Can you work these out from the drawing? Everything is in mm from the part's minimum corner. A direction names the side the tool comes from. Give positions to 0.01 mm unless a question says otherwise; leave off trailing zeros. Write each loop counter-clockwise with the first axis right and the second up, starting at its lowest first coordinate (ties: lowest second). Pieces come first, ordered by that corner, then holes. Notation, with made-up numbers: M 45.5,-20.75 L 70.5,-20.75 A28 ccw 70.5,18.25 Z; hole C -20,-17.75 d1. An arc over 180 degrees is marked long. One line per item, written item: value.
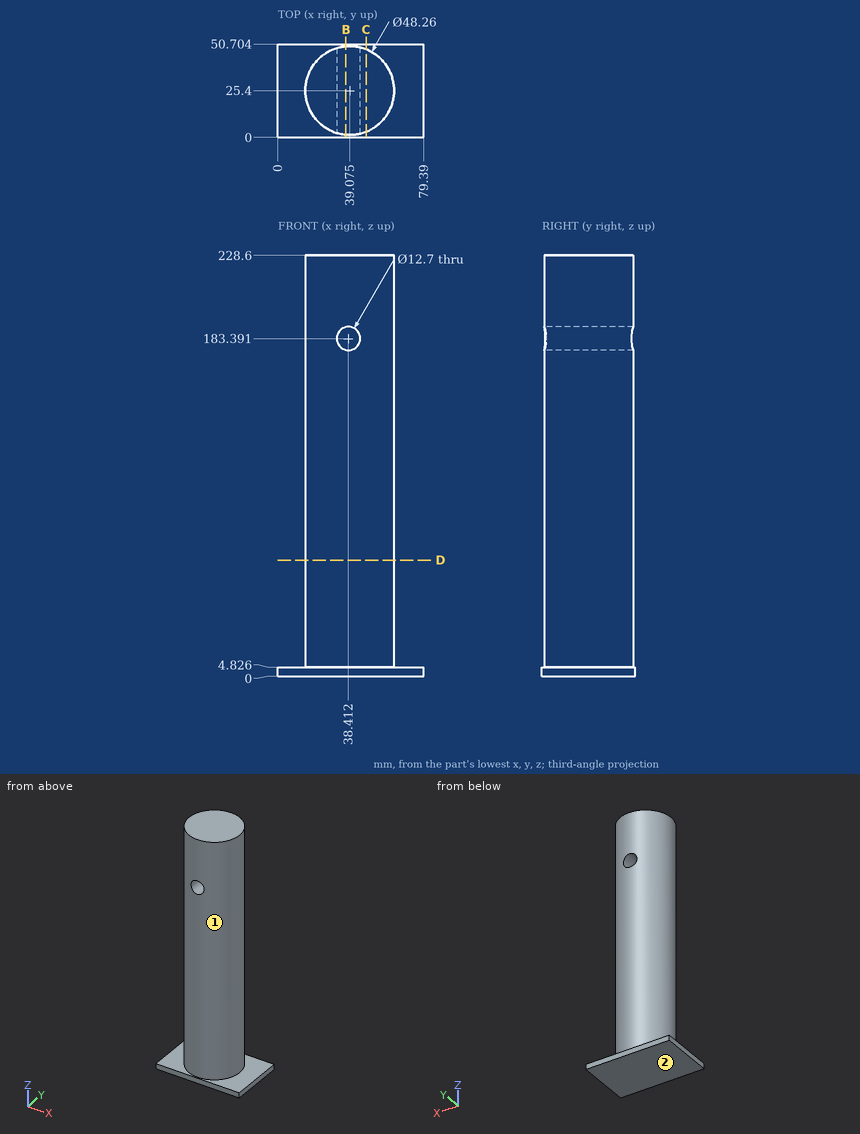
1) I'm going to push flat-ended pins straight in: pin 1 (6 mm diameter, centred on y = 19.5, z = 107, fed in from -X); pin 2 (14.5 mm diameter, centred on x = 38.41, z = 183.39, fed in from -Y); pin 3 (4 mm diameter, centred on x = 56.5, z = 78, fed in from +Y) (1 decimal); pin 4 (4 mm diameter, centred on x = 12.5, y = 25, fed in from -Z). Where does each tip first touch, or does it pass through?
Outcome:
pin 1: stops at x = 15.12
pin 2: stops at y = 1.27
pin 3: stops at y = 44
pin 4: stops at z = 0
2) If we section it at D-D, the plane z = 63: Write out the boundary of the cut face in (x, y) (1 decimal), then the cut area to 3 significant figures.
Outcome:
outline: C 39.1,25.4 d48.3
area: 1,830 mm^2
3) If we section it at B-B, the plane x = 37: Write out the boundary of the cut face in (y, z), then the cut area to 3 significant figures.
Outcome:
outline: M 0,0 L 50.7,0 L 50.7,4.83 L 49.44,4.83 L 49.44,177.2 L 1.36,177.2 L 1.36,4.83 L 0,4.83 Z; M 1.36,189.58 L 49.44,189.58 L 49.44,228.6 L 1.36,228.6 Z
area: 10,400 mm^2
4) If we section it at C-C, the plane x = 48: Write out the boundary of the cut face in (y, z), then the cut area to 3 significant figures.
Outcome:
outline: M 0,0 L 50.7,0 L 50.7,4.83 L 47.82,4.83 L 47.82,228.6 L 2.98,228.6 L 2.98,4.83 L 0,4.83 Z
area: 10,300 mm^2
5) Please list where these lines run through material, in increasing order: L1, parallel to Z at x = 36.5, y = 24 (1 decimal); L2, parallel to Z at x = 64, y = 11; L3, parallel to X at y = 9, z = 188.5 (1 decimal). Write a range as from..to.
Outcome:
L1: z = 0..177.3, 189.4..228.6
L2: z = 0..4.83
L3: x = 21.4..34.6, 42.2..56.8
6) On a 3-axis mill with a long thin cutter (end or side, diameter ignored), from which of +Z, -Z, +X, -X, +Y, -Y can I reach the whole of each face in a straight line? I mean the marked faces 1 and 2. Say none if no direction works.
Outcome:
face 1: +Z
face 2: -Z, +X, -X, +Y, -Y
